The figure shows three views and two pictorial views of one solid part (mm, origin at its lowest corner). Answer the questions. Coordinates: 2 decimals unless noted, no trailing zeros. Loops run counter-clockwise (first coordinate to the right, second up) from the corner with the lowest first, then second, coordinate; pieces in that order, holes last. Notation, with made-up numbers: (14.25, -23.5) - (67.25, -23.5) arc R28 cw to (67.25, 2.5) - close; hole circle Ø8 at (4.5, 83). An arc over 180 degrees is marked (long way). One line per question, with ' | ' between items.
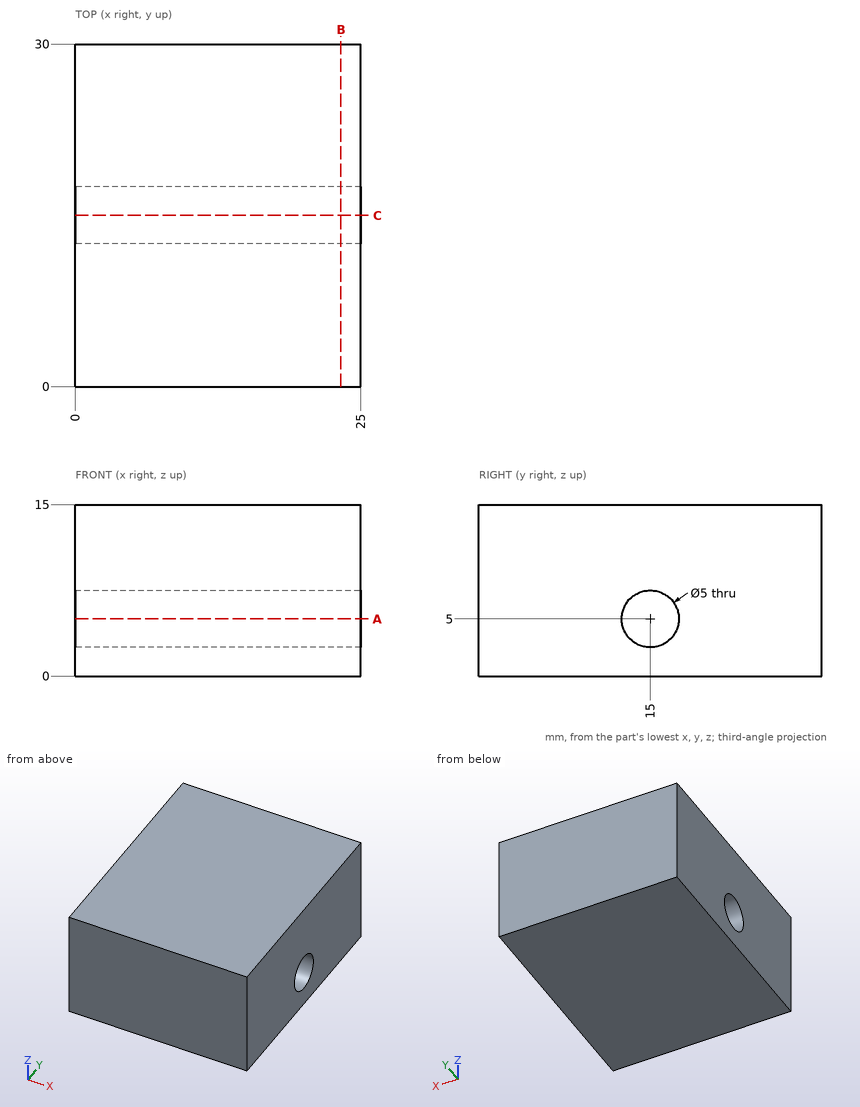
Item 1: Find section C-C, the plane y = 15. Write down the section's boundary in (x, z), plus the area to 3 significant figures.
Taken from the geometry:
outline: (0, 0) - (25, 0) - (25, 2.5) - (0, 2.5) - close; (0, 7.5) - (25, 7.5) - (25, 15) - (0, 15) - close | area: 250 mm2
Item 2: Find the intervals of material crossed by line 1 (Y direction, x = 9.25, z = 5); line 2 (Y direction, x = 24, z = 6.5); line 3 (Z direction, x = 9, y = 14.5), in increasing order. Write a range as [from, to].
Taken from the geometry:
line 1: y = [0, 12.5], [17.5, 30] | line 2: y = [0, 13], [17, 30] | line 3: z = [0, 2.55], [7.45, 15]
Item 3: Find section B-B, the plane x = 23.25. Write down the section's boundary in (y, z), plus the area to 3 significant figures.
Taken from the geometry:
outline: (0, 0) - (30, 0) - (30, 15) - (0, 15) - close; hole circle Ø5 at (15, 5) | area: 430 mm2
Item 4: Find section A-A, the plane z = 5. Write down the section's boundary in (x, y).
Taken from the geometry:
outline: (0, 0) - (25, 0) - (25, 12.5) - (0, 12.5) - close; (0, 17.5) - (25, 17.5) - (25, 30) - (0, 30) - close
